Here's how the part is built. I have some questions about the finished solid (model axes, mm). Face numbers are marked on the shaded views. A direction names the side the tool comes from. Coordinates: 2 decimals unless noted, no trailing zeros. Order: outer loops, then holes, each group sorted by start corner. A loop starts at its lowest first (then second) coordinate and runs counter-clockwise, first axis right, second up. Notation, with made-up numbers: (46.25, 19.25) - (66.25, 19.25) arc R34 cw to (66.25, 52.25) - close; hole circle Ø9 at (41, 62). An arc over 180 degrees is marked (long way). Answer in a Markdown table with one row per item. Add a question column.
Item 1: I want a section at B-B (z = -2.75). Count the separate pieces of the cut face and the enclosed holes in it, plus the area to 3 significant figures.
Item 2: Will these pins go through, and if not, where does the flat tip stop? pin 1 Ø1.5 at (x, y) = (26, 10.5) entering from -Z; pin 2 Ø3.5 at (y, z) = (12, 2.5) entering from -X; pin 3 Ø12 at (x, y) = (-26.5, 1) entering from +Z.
Item 3: I want a section at A-A (x = 12.5). Please give me the cut outline in (y, z), plus the area to 3 significant figures.
Item 4: Thinking about a two-plate mould opening in X: for the marked faces 5 and 6, which applies, +X half, -X half, draft (parallel to the pull), parting line (faces both ways), or undercut?
Item 5: On a 3-axis mill with a long thin cutter (end or side, diameter ignored), from which of +Z, -Z, +X, -X, +Y, -Y can I reach the whole of each face in a straight line? I mean the marked faces 1, 2, 3 and 4. Say none if no direction works.
Item 6: I want a section at C-C (y = 2). Please give me the cut outline in (x, z).
Item 7: I want a section at D-D (x = -7). Please give me the cut outline in (y, z).
Item 8: If I drill on line 1 along X through (y, z) = (-2.75, 0.5); line 2 along X through (y, z) = (5.25, 0.75); line 3 along X through (y, z) = (4.75, -3.5), over which ranges is the centre line in solid material (lowest first)? Write a range as from..to.
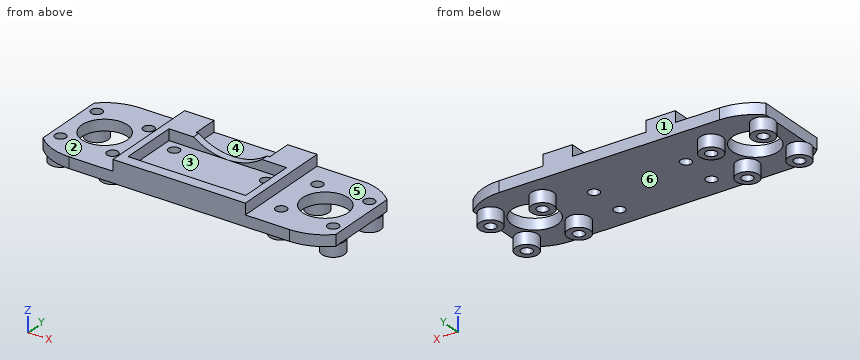
```python
from build123d import *

# Parameters (mm, degrees)
SKETCH1_R              = 6.2
MAIN_DEPTH             = 1.5
SKETCH2_W              = 32
SKETCH2_H              = 16
FRAMEWORK_DEPTH        = 3
SKETCH3_R              = 1.5
FIXHOLE_DEPTH          = 7
HOLEPATTERN_COUNT      = 2
HOLEPATTERN_PITCH      = 25
HOLEPATTERN_COUNT_DIR2 = 2
HOLEPATTERN_PITCH_DIR2 = 10
SKETCH4_R              = 3.05
SKETCH4_R_2            = 1.5
FORLMK6UU_DEPTH        = 3.3
SKETCH5_R              = 1.5
CUT_EXTRUDE1_DEPTH     = 7.3
SKETCH6_R              = 16
CUT_EXTRUDE2_DEPTH     = 2


with BuildPart() as part:
    # Sketch1 → Main (new body, symmetric)
    with BuildSketch(Plane.XY):
        with BuildLine():
            Line((-39.8, 9.9979998), (-39.8, -9.9979998))
            ThreePointArc((-39.8, -9.9979998), (-35.292825465, -12.96094127), (-30, -14))
            Line((-30, -14), (30, -14))
            ThreePointArc((30, -14), (35.292825465, -12.96094127), (39.8, -9.9979998))
            Line((39.8, -9.9979998), (39.8, 9.9979998))
            ThreePointArc((39.8, 9.9979998), (35.292825465, 12.96094127), (30, 14))
            Line((30, 14), (-30, 14))
            ThreePointArc((-30, 14), (-35.292825465, 12.96094127), (-39.8, 9.9979998))
        make_face()
        with Locations((-30, 0)):
            Circle(SKETCH1_R, mode=Mode.SUBTRACT)
        with Locations((30, 0)):
            Circle(SKETCH1_R, mode=Mode.SUBTRACT)
    extrude(amount=MAIN_DEPTH, both=True)

    # Sketch2 → Framework (add)
    with BuildSketch(Plane(origin=(0, 0, 1.5), x_dir=(-1, 0, 0), z_dir=(0, 0, -1))):
        Polygon((18, 14), (10, 14), (10, 7), (-10, 7), (-10, 14), (-18, 14), (-18, -14), (18, -14), align=None)
        with Locations((0, -3)):
            Rectangle(SKETCH2_W, SKETCH2_H, mode=Mode.SUBTRACT)
    extrude(amount=-FRAMEWORK_DEPTH)

    # Sketch3 → FixHole (cut, through all)
    with BuildSketch(Plane(origin=(0, 0, -1.5), x_dir=(-1, 0, 0), z_dir=(0, 0, -1))):
        with Locations((12.5, -8)):
            Circle(SKETCH3_R)
    fixhole = extrude(amount=-FIXHOLE_DEPTH, mode=Mode.SUBTRACT)

    # HolePattern: FixHole 2 × 2
    with Locations(*[(i * HOLEPATTERN_PITCH, j * HOLEPATTERN_PITCH_DIR2, 0) for i in range(HOLEPATTERN_COUNT) for j in range(HOLEPATTERN_COUNT_DIR2) if (i, j) != (0, 0)]):
        add(fixhole, mode=Mode.SUBTRACT)

    # Sketch4 → ForLMK6UU (add)
    with BuildSketch(Plane.XY.offset(-1.5)):
        with Locations((-37.071067812, 7.071067812)):
            Circle(SKETCH4_R)
        with Locations((-37.071067812, 7.071067812)):
            Circle(SKETCH4_R_2, mode=Mode.SUBTRACT)
        with Locations((-22.928932188, -7.071067812)):
            Circle(SKETCH4_R)
        with Locations((-22.928932188, -7.071067812)):
            Circle(SKETCH4_R_2, mode=Mode.SUBTRACT)
        with Locations((-22.928932188, 7.071067812)):
            Circle(SKETCH4_R)
        with Locations((-22.928932188, 7.071067812)):
            Circle(SKETCH4_R_2, mode=Mode.SUBTRACT)
        with Locations((-37.071067812, -7.071067812)):
            Circle(SKETCH4_R)
        with Locations((-37.071067812, -7.071067812)):
            Circle(SKETCH4_R_2, mode=Mode.SUBTRACT)
    forlmk6uu = extrude(amount=-FORLMK6UU_DEPTH)

    # Sketch5 → Cut-Extrude1 (cut, through all)
    with BuildSketch(Plane.XY.offset(1.5)):
        with Locations((-37.071067812, 7.071067812)):
            Circle(SKETCH5_R)
        with Locations((-22.928932188, 7.071067812)):
            Circle(SKETCH5_R)
        with Locations((-37.071067812, -7.071067812)):
            Circle(SKETCH5_R)
        with Locations((-22.928932188, -7.071067812)):
            Circle(SKETCH5_R)
    cut_extrude1 = extrude(amount=-CUT_EXTRUDE1_DEPTH, mode=Mode.SUBTRACT)

    # Mirror1: ForLMK6UU, Cut-Extrude1 across plane
    add(forlmk6uu.mirror(Plane(origin=(0, 0, 0), x_dir=(0, 0, 1), z_dir=(1, 0, 0))))
    add(cut_extrude1.mirror(Plane(origin=(0, 0, 0), x_dir=(0, 0, 1), z_dir=(1, 0, 0))), mode=Mode.SUBTRACT)

    # Sketch6 → Cut-Extrude2 (cut)
    with BuildSketch(Plane(origin=(0, 7, 0), x_dir=(1, 0, 0), z_dir=(0, 1, 0))):
        with Locations((0, -17.5)):
            Circle(SKETCH6_R)
    extrude(amount=-CUT_EXTRUDE2_DEPTH, mode=Mode.SUBTRACT)


solid = part.part
```
Values follow:
| question | item | result |
|---|---|---|
| 1 | separate pieces | 8 |
| 1 | enclosed holes | 8 |
| 1 | area | 177 mm^2 |
| 2 | pin 1 | stops at z = -1.5 |
| 2 | pin 2 | stops at x = -39.19 |
| 2 | pin 3 | stops at z = 1.5 |
| 3 | outline | (-14, -1.5) - (-9.5, -1.5) - (-9.5, 1.5) - (-11, 1.5) - (-11, 4.5) - (-14, 4.5) - close; (-6.5, -1.5) - (0.5, -1.5) - (0.5, 1.5) - (-6.5, 1.5) - close; (3.5, -1.5) - (14, -1.5) - (14, 4.5) - (5, 4.5) - (5, 1.5) - (3.5, 1.5) - close |
| 3 | area | 102 mm^2 |
| 4 | face 5 | draft |
| 4 | face 6 | undercut |
| 5 | face 1 | +Z, -Z, +X, -X, +Y |
| 5 | face 2 | +Z, -X, +Y, -Y |
| 5 | face 3 | +Z |
| 5 | face 4 | +Z, +Y |
| 6 | outline | (-39.8, -1.5) - (-35.87, -1.5) - (-35.87, 1.5) - (-39.8, 1.5) - close; (-24.13, -1.5) - (-14, -1.5) - (-14, 1.5) - (-16, 1.5) - (-16, 4.5) - (-18, 4.5) - (-18, 1.5) - (-24.13, 1.5) - close; (-11, -1.5) - (11, -1.5) - (11, 1.5) - (-11, 1.5) - close; (14, -1.5) - (24.13, -1.5) - (24.13, 1.5) - (18, 1.5) - (18, 4.5) - (16, 4.5) - (16, 1.5) - (14, 1.5) - close; (35.87, -1.5) - (39.8, -1.5) - (39.8, 1.5) - (35.87, 1.5) - close |
| 7 | outline | (-14, -1.5) - (14, -1.5) - (14, 1.5) - (7, 1.5) - (7, 3.11) - (5, 3.11) - (5, 1.5) - (-11, 1.5) - (-11, 4.5) - (-14, 4.5) - close |
| 8 | line 1 | x = -39.8..-35.56, -24.44..24.44, 35.56..39.8 |
| 8 | line 2 | x = -39.8..-33.3, -26.7..26.7, 33.3..39.8 |
| 8 | line 3 | x = -39.05..-35.09, -24.91..-20.95, 20.95..24.91, 35.09..39.05 |
